Geometry check sheet. Reference: the model listing, model coordinates, mm. A direction names the side the tool comes from. Coordinates: 2 decimals unless noted, no trailing zeros. Write each loop counter-clockwise with the first axis right and the second up, starting at its lowest first coordinate (ties: lowest second). Pieces come first, ordered by that corner, then holes. Notation, with made-up numbers: (54, 82) - (70, 82) arc R21 cw to (70, 118) - close; hole circle Ø8 at (53.25, 76). An arc over 180 degrees is marked (long way). Answer as a JSON object with one key per item and string values. Group by question number.
from build123d import *

# Parameters (mm, degrees)
SKETCH1_W           = 1310
SKETCH1_H           = 2070
BOSS_EXTRUDE1_DEPTH = 400
SKETCH2_W           = 1200
SKETCH2_H           = 400
CUT_EXTRUDE2_DEPTH  = 397
SKETCH5_W           = 1200
SKETCH5_H           = 10
CUT_EXTRUDE5_DEPTH  = 397
SKETCH6_W           = 1200
SKETCH6_H           = 10
CUT_EXTRUDE6_DEPTH  = 397
LPATTERN2_COUNT     = 3
LPATTERN2_PITCH     = 200
SKETCH9_W           = 100
SKETCH9_H           = 30
BOSS_EXTRUDE2_DEPTH = 10
LPATTERN3_COUNT     = 4
LPATTERN3_PITCH     = 200
SKETCH11_W          = 110
SKETCH11_H          = 2070
BOSS_EXTRUDE3_DEPTH = 400
SKETCH12_W          = 500
SKETCH12_H          = 10
CUT_EXTRUDE9_DEPTH  = 397
SKETCH13_W          = 1200
SKETCH13_H          = 870
CUT_EXTRUDE10_DEPTH = 397
SKETCH14_W          = 500
SKETCH14_H          = 10
BOSS_EXTRUDE4_DEPTH = 397
LPATTERN4_COUNT     = 2
LPATTERN4_PITCH     = 385
SKETCH16_W          = 5
SKETCH16_H          = 780
CUT_EXTRUDE11_DEPTH = 397
SKETCH17_W          = 450
SKETCH17_H          = 800
BOSS_EXTRUDE5_DEPTH = 397


with BuildPart() as part:
    # Sketch1 → Boss-Extrude1 (new body)
    with BuildSketch(Plane.XY):
        Rectangle(SKETCH1_W, SKETCH1_H)
    extrude(amount=BOSS_EXTRUDE1_DEPTH)

    # Sketch2 → Cut-Extrude2 (cut)
    with BuildSketch(Plane.XY.offset(400)):
        with Locations((-55, -35)):
            Rectangle(SKETCH2_W, SKETCH2_H)
    extrude(amount=-CUT_EXTRUDE2_DEPTH, mode=Mode.SUBTRACT)

    # Sketch5 → Cut-Extrude5 (cut)
    with BuildSketch(Plane.XY.offset(400)):
        with Locations((-55, -250)):
            Rectangle(SKETCH5_W, SKETCH5_H)
    extrude(amount=-CUT_EXTRUDE5_DEPTH, mode=Mode.SUBTRACT)

    # Sketch6 → Cut-Extrude6 (cut)
    with BuildSketch(Plane.XY.offset(400)):
        with Locations((-55, -460)):
            Rectangle(SKETCH6_W, SKETCH6_H)
    cut_extrude6 = extrude(amount=-CUT_EXTRUDE6_DEPTH, mode=Mode.SUBTRACT)

    # LPattern2: Cut-Extrude6 ×3
    with Locations(*[(0, -i * LPATTERN2_PITCH, 0) for i in range(1, LPATTERN2_COUNT)]):
        add(cut_extrude6, mode=Mode.SUBTRACT)

    # Sketch9 → Boss-Extrude2 (add)
    with BuildSketch(Plane.XY.offset(400)):
        with Locations((-55, -304.237135846)):
            Rectangle(SKETCH9_W, SKETCH9_H)
    boss_extrude2 = extrude(amount=BOSS_EXTRUDE2_DEPTH)

    # LPattern3: Boss-Extrude2 ×4
    with Locations(*[(0, -i * LPATTERN3_PITCH, 0) for i in range(1, LPATTERN3_COUNT)]):
        add(boss_extrude2)

    # Sketch12 → Cut-Extrude9 (cut)
    with BuildSketch(Plane.XY.offset(400)):
        with Locations((295, 670)):
            Rectangle(SKETCH12_W, SKETCH12_H)
    extrude(amount=-CUT_EXTRUDE9_DEPTH, mode=Mode.SUBTRACT)

    # Sketch13 → Cut-Extrude10 (cut)
    with BuildSketch(Plane.XY.offset(400)):
        with Locations((-55, 600)):
            Rectangle(SKETCH13_W, SKETCH13_H)
    extrude(amount=-CUT_EXTRUDE10_DEPTH, mode=Mode.SUBTRACT)



with BuildPart() as body_2:
    # Sketch11 → Boss-Extrude3 (new body)
    with BuildSketch(Plane.XY.offset(400)):
        with Locations((600, 0)):
            Rectangle(SKETCH11_W, SKETCH11_H)
    extrude(amount=-BOSS_EXTRUDE3_DEPTH)


with BuildPart() as part_1:
    add(part.part)

    add(body_2.part)  # Boss-Extrude4 merges body 2
    # Sketch14 → Boss-Extrude4 (add)
    with BuildSketch(Plane.XY.offset(3)):
        with Locations((295, 155)):
            Rectangle(SKETCH14_W, SKETCH14_H)
    boss_extrude4 = extrude(amount=BOSS_EXTRUDE4_DEPTH)

    # LPattern4: Boss-Extrude4 ×2
    with Locations(*[(0, i * LPATTERN4_PITCH, 0) for i in range(1, LPATTERN4_COUNT)]):
        add(boss_extrude4)

    # Sketch16 → Cut-Extrude11 (cut)
    with BuildSketch(Plane.XY.offset(400)):
        with Locations((542.5, -645)):
            Rectangle(SKETCH16_W, SKETCH16_H)
    extrude(amount=-CUT_EXTRUDE11_DEPTH, mode=Mode.SUBTRACT)

    # Sketch17 → Boss-Extrude5 (add)
    with BuildSketch(Plane.XY.offset(3)):
        with Locations((-290, 400)):
            Rectangle(SKETCH17_W, SKETCH17_H)
    extrude(amount=BOSS_EXTRUDE5_DEPTH)


solid = part_1.part
(1) Draft check along X on faces 5 (the face through (292, 160, 199)), 6 (the face through (292, 535, 199)), 7 (the face through (-66, -455, 204)). Enter one of: +X half, -X half, draft (parallel to the pull), parting line (faces both ways), or undercut.
(2) Set-up check for faces 1 (the face through (292, 545, 199)), 2 (the face through (545, 345, 204)), 3 (the face through (540, -356, 204)), 4 (the face through (-63, -235, 204)): record each of +Z, -Z, +X, -X, +Y, -Y from which the full face is reachable in a straight line by a thin tool's end or side.
(3) Section check B-B (y = -573.5). Record the cut outline in (x, z), and give its area (3 significant figures).
(4) Gauge pin test, flat ends, axial feed: pin 1 (3 mm diameter, centred on x = -68.5, z = 404.5, fed in from -Y); pin 2 (8 mm diameter, centred on y = 155.5, z = 179.5, fed in from -X); pin 3 (4 mm diameter, centred on x = 363, y = -607, fed in from +Z). Record the tip position at first contact, or that the pin passes through.
(5) Section check C-C (z = 252.5). Count the separate pieces of the cut face and the enclosed holes in it, and give its area (3 significant figures).
(6) Section check A-A (x = -397). Record the cut outline in (y, z), and give its area (3 significant figures).
(7) Material ranges on L1, parallel to Y at x = -182.5, z = 287; L2, parallel to Y at x = 34, z = 274; L3, parallel to X at y = 587, z = 341.5, recorded low to high. Write a range as [from, to].
Conclusion:
{
 "1": {"face 5": "undercut", "face 6": "undercut", "face 7": "draft"},
 "2": {"face 1": "+Z, +Y", "face 2": "+Z", "face 3": "+Z, -Y", "face 4": "+Z, -X"},
 "3": {"outline": "(-655, 0) - (655, 0) - (655, 400) - (545, 400) - (545, 3) - (540, 3) - (540, 400) - (-655, 400) - close", "area": "522,000 mm^2"},
 "4": {"pin 1": "stops at y = -919.24", "pin 2": "stops at x = -515", "pin 3": "stops at z = 400"},
 "5": {"separate pieces": "6", "enclosed holes": "0", "area": "1,510,000 mm^2"},
 "6": {"outline": "(-1035, 0) - (1035, 0) - (1035, 3) - (800, 3) - (800, 400) - (0, 400) - (0, 3) - (-235, 3) - (-235, 400) - (-245, 400) - (-245, 3) - (-255, 3) - (-255, 400) - (-455, 400) - (-455, 3) - (-465, 3) - (-465, 400) - (-655, 400) - (-655, 3) - (-665, 3) - (-665, 400) - (-855, 400) - (-855, 3) - (-865, 3) - (-865, 400) - (-1035, 400) - close", "area": "626,000 mm^2"},
 "7": {"L1": "y = [-1035, -865], [-855, -665], [-655, -465], [-455, -255], [-245, -235], [0, 800]", "L2": "y = [-1035, -865], [-855, -665], [-655, -465], [-455, -255], [-245, -235]", "L3": "x = [-515, -65], [545, 655]"}
}
